from build123d import *

# Parameters (mm, degrees)
EXTRUDE_1_DEPTH = 30
FILLET_1_R      = 0.3


with BuildPart() as part:
    # Эскиз1 → Бобышка-Вытянуть1 (new body)
    with BuildSketch(Plane.XY):
        with BuildLine():
            Line((21.5, 0), (-21.5, 0))
            Line((-21.5, 0), (-21.5, 19.5))
            ThreePointArc((-21.5, 19.5), (-21, 20), (-20.5, 19.5))
            Line((-20.5, 19.5), (-20.5, 5))
            Line((-20.5, 5), (-19.95, 5))
            Line((-19.95, 5), (-19.95, 3.836660027))
            ThreePointArc((-19.95, 3.836660027), (-19.5, 2.05), (-19.05, 3.836660027))
            Line((-19.05, 3.836660027), (-19.05, 5))
            Line((-19.05, 5), (-17.4, 5))
            Line((-17.4, 5), (-17.4, 3))
            Line((-17.4, 3), (-15.5, 3))
            Line((-15.5, 3), (-15.5, 19.5))
            ThreePointArc((-15.5, 19.5), (-15, 20), (-14.5, 19.5))
            Line((-14.5, 19.5), (-14.5, 2))
            Line((-14.5, 2), (-9.5, 2))
            Line((-9.5, 2), (-9.5, 19.5))
            ThreePointArc((-9.5, 19.5), (-9, 20), (-8.5, 19.5))
            Line((-8.5, 19.5), (-8.5, 2))
            Line((-8.5, 2), (-3.5, 2))
            Line((-3.5, 2), (-3.5, 19.5))
            ThreePointArc((-3.5, 19.5), (-3, 20), (-2.5, 19.5))
            Line((-2.5, 19.5), (-2.5, 2))
            Line((-2.5, 2), (2.5, 2))
            Line((2.5, 2), (2.5, 19.5))
            ThreePointArc((2.5, 19.5), (3, 20), (3.5, 19.5))
            Line((3.5, 19.5), (3.5, 2))
            Line((3.5, 2), (8.5, 2))
            Line((8.5, 2), (8.5, 19.5))
            ThreePointArc((8.5, 19.5), (9, 20), (9.5, 19.5))
            Line((9.5, 19.5), (9.5, 2))
            Line((9.5, 2), (14.5, 2))
            Line((14.5, 2), (14.5, 19.5))
            ThreePointArc((14.5, 19.5), (15, 20), (15.5, 19.5))
            Line((15.5, 19.5), (15.5, 3))
            Line((15.5, 3), (17.4, 3))
            Line((17.4, 3), (17.4, 5))
            Line((17.4, 5), (19.05, 5))
            Line((19.05, 5), (19.05, 3.836660027))
            ThreePointArc((19.05, 3.836660027), (19.5, 2.05), (19.95, 3.836660027))
            Line((19.95, 3.836660027), (19.95, 5))
            Line((19.95, 5), (20.5, 5))
            Line((20.5, 5), (20.5, 19.5))
            ThreePointArc((20.5, 19.5), (21, 20), (21.5, 19.5))
            Line((21.5, 19.5), (21.5, 0))
        make_face()
    extrude(amount=EXTRUDE_1_DEPTH)

    # Скругление1
    fillet_1_edges = [part.edges().sort_by_distance(p)[0] for p in [
        (-19.95, 5, 15),
        (-19.05, 5, 15),
        (-17.4, 5, 15),
        (17.4, 5, 15),
        (19.05, 5, 15),
        (19.95, 5, 15),
    ]]
    fillet(fillet_1_edges, radius=FILLET_1_R)


solid = part.part
CAD build for the part. Positions are in the model's coordinates, mm. A direction names the side the tool comes from. Coordinates: 2 decimals unless noted, no trailing zeros. Order: outer loops, then holes, each group sorted by start corner. A loop starts at its lowest first (then second) coordinate and runs counter-clockwise, first axis right, second up.
Item 1: Two-plate mould, pull along X, no slides. Class faces 1 (the face through (-3.5, 11, 15)), 2 (the face through (21.5, 10, 15)): +X half, -X half, draft (parallel to the pull), parting line (faces both ways), or undercut.
Check sheet entries:
face 1: undercut
face 2: +X half
Item 2: Band-saw the part on B-B on x = 8. List the corners of the cut face in (y, z), plus the area to 3 significant figures.
Check sheet entries:
outline: (0, 0) - (2, 0) - (2, 30) - (0, 30) - close
area: 60.0 mm2
Item 3: Band-saw the part on C-C on x = 19.5. List the corners of the cut face in (y, z).
Check sheet entries:
outline: (0, 0) - (2.05, 0) - (2.05, 30) - (0, 30) - close
Item 4: 3-axis set-ups, long thin cutter, end or side, ignore diameter. For faces 3 (the face through (-19.54, 2.05, 14.79)), 4 (the face through (17.4, 4, 15)): which of +Z, -Z, +X, -X, +Y, -Y reach the whole face in a straight line?
Check sheet entries:
face 3: +Z, -Z
face 4: +Z, -Z, +Y
Item 5: Pin check, flat tips, straight feed: pin 1 Ø1.5 at (x, z) = (-5, 19) entering from +Y; pin 2 Ø3 at (x, y) = (15, 6) entering from -Z; pin 3 Ø0.6 at (x, z) = (16, 19.5) entering from +Y. Stop position of each tip, or through.
Check sheet entries:
pin 1: stops at y = 2
pin 2: stops at z = 0
pin 3: stops at y = 3
Item 6: Band-saw the part on A-A on y = 18.5. Give the number of separate pieces and of enclosed holes in the cut face, plus the area to 3 significant figures.
Check sheet entries:
separate pieces: 8
enclosed holes: 0
area: 240 mm2
Item 7: Drill centre lines: L1, parallel to Y at x = 12.5, z = 4.5; L2, parallel to Y at x = -19.5, z = 7.5. Where is each one in solid material? Low to high.
Check sheet entries:
L1: y = 0 to 2
L2: y = 0 to 2.05
